from build123d import *

# Parameters (mm, degrees)
BOSS_EXTRUDE1_DEPTH       = 80
SKETCH2_W                 = 60
SKETCH2_H                 = 80
BOSS_EXTRUDE6_DEPTH       = 10
CUT_EXTRUDE3_DEPTH        = 149
BOSS_EXTRUDE7_DEPTH       = 20
SKETCH11_W                = 100
SKETCH11_H                = 80
CUT_EXTRUDE4_DEPTH        = 20
CUT_EXTRUDE5_DEPTH        = 20
SKETCH14_W                = 24.037008503
SKETCH14_H                = 50
CUT_EXTRUDE6_DEPTH        = 29
SKETCH15_W                = 46.666666667
SKETCH15_H                = 50
CUT_EXTRUDE7_DEPTH        = 29
SKETCH16_W                = 20
SKETCH16_H                = 30
BOSS_EXTRUDE8_DEPTH       = 70
BOSS_EXTRUDE10_DEPTH      = 30
SKETCH21_W                = 43.205783384
SKETCH21_H                = 74.052806938
CUT_EXTRUDE9_DEPTH        = 30
SKETCH22_W                = 30
SKETCH22_H                = 20
CUT_EXTRUDE10_DEPTH       = 30
BOSS_EXTRUDE11_DEPTH      = 30
BOSS_EXTRUDE12_DEPTH      = 40
BOSS_EXTRUDE12_DEPTH_BACK = 30
SKETCH25_W                = 50
SKETCH25_H                = 20
BOSS_EXTRUDE13_DEPTH      = 60
BOSS_EXTRUDE16_DEPTH      = 50
BOSS_EXTRUDE17_DEPTH      = 20


with BuildPart() as part:
    # Sketch1 → Boss-Extrude1 (new body)
    with BuildSketch(Plane(origin=(0, 0, 0), x_dir=(1, 0, 0), z_dir=(0, 1, 0))):
        Polygon((0, 0), (0, 60), (40, 60), (40, 30), (30, 30), (30, 20), align=None)
    extrude(amount=BOSS_EXTRUDE1_DEPTH)

    # Sketch2 → Boss-Extrude6 (add)
    with BuildSketch(Plane.ZY):
        with Locations((-30, 40)):
            Rectangle(SKETCH2_W, SKETCH2_H)
        Polygon((40, 0), (0, 0), (0, 80), (20, 50), (40, 50), align=None)
    extrude(amount=-BOSS_EXTRUDE6_DEPTH)

    # Sketch8 → Cut-Extrude3 (cut)
    with BuildSketch(Plane(origin=(18.823529412, 18.823529412, 28.235294118), x_dir=(0.874474632, -0.269069118, -0.403603676), z_dir=(0.48507125, 0.48507125, 0.727606875))):
        Polygon((-21.525529408, 30.508510792), (12.780783086, 41.602514717), (12.780783086, 77.658027472), (-21.525529408, 66.564023547), align=None)
    extrude(amount=CUT_EXTRUDE3_DEPTH, mode=Mode.SUBTRACT)

    # Sketch10 → Boss-Extrude7 (add)
    with BuildSketch(Plane(origin=(18.823529412, 18.823529412, 28.235294118), x_dir=(0.874474632, -0.269069118, -0.403603676), z_dir=(0.48507125, 0.48507125, 0.727606875))):
        Polygon((-21.525529408, 30.508510792), (12.780783086, 41.602514717), (12.780783086, 77.658027472), (-21.525529408, 66.564023547), align=None)
    extrude(amount=-BOSS_EXTRUDE7_DEPTH)

    # Sketch11 → Cut-Extrude4 (cut)
    with BuildSketch(Plane.ZY):
        with Locations((-10, 40)):
            Rectangle(SKETCH11_W, SKETCH11_H)
    extrude(amount=CUT_EXTRUDE4_DEPTH, mode=Mode.SUBTRACT)

    # Sketch12 → Cut-Extrude5 (cut)
    with BuildSketch(Plane(origin=(0, 50, 0), x_dir=(1, 0, 0), z_dir=(0, 1, 0))):
        Polygon((0, -20), (10, -13.333333333), (10, -40), (0, -40), align=None)
    extrude(amount=CUT_EXTRUDE5_DEPTH, mode=Mode.SUBTRACT)

    # Sketch14 → Cut-Extrude6 (cut)
    with BuildSketch(Plane(origin=(0, 0, 0), x_dir=(0.832050294, 0, -0.554700196), z_dir=(0.554700196, 0, 0.832050294))):
        with Locations((24.037008504, 25)):
            Rectangle(SKETCH14_W, SKETCH14_H)
    extrude(amount=CUT_EXTRUDE6_DEPTH, mode=Mode.SUBTRACT)

    # Sketch15 → Cut-Extrude7 (cut)
    with BuildSketch(Plane(origin=(10, 0, 0), x_dir=(0, 0, -1), z_dir=(1, 0, 0))):
        with Locations((-16.666666666, 25)):
            Rectangle(SKETCH15_W, SKETCH15_H)
    extrude(amount=CUT_EXTRUDE7_DEPTH, mode=Mode.SUBTRACT)

    # Sketch16 → Boss-Extrude8 (add)
    with BuildSketch(Plane(origin=(0, 70, 0), x_dir=(1, 0, 0), z_dir=(0, 1, 0))):
        with Locations((50, 45)):
            Rectangle(SKETCH16_W, SKETCH16_H)
    extrude(amount=-BOSS_EXTRUDE8_DEPTH)

    # Sketch17 → Boss-Extrude10 (add)
    with BuildSketch(Plane(origin=(0, 0, -60), x_dir=(-1, 0, 0), z_dir=(0, 0, -1))):
        Polygon((-80, 10), (-80, 0), (-60, 0), (-60, 70), (-100, 10), align=None)
    extrude(amount=-BOSS_EXTRUDE10_DEPTH)

    # Sketch21 → Cut-Extrude9 (cut)
    with BuildSketch(Plane.XY.offset(-30)):
        with Locations((81.602891692, 32.973596531)):
            Rectangle(SKETCH21_W, SKETCH21_H)
    extrude(amount=-CUT_EXTRUDE9_DEPTH, mode=Mode.SUBTRACT)

    # Sketch22 → Cut-Extrude10 (cut)
    with BuildSketch(Plane.XY.offset(-30)):
        with Locations((45, 10)):
            Rectangle(SKETCH22_W, SKETCH22_H)
    extrude(amount=-CUT_EXTRUDE10_DEPTH, mode=Mode.SUBTRACT)

    # Sketch23 → Boss-Extrude11 (add)
    with BuildSketch(Plane.XY.offset(-30)):
        Polygon((60, 70), (100, 30), (80, 30), (80, 20), (60, 20), align=None)
    extrude(amount=-BOSS_EXTRUDE11_DEPTH)

    # Sketch24 → Boss-Extrude12 (add, two sides)
    with BuildSketch(Plane.XY.offset(-30)) as boss_extrude12_sk:
        Polygon((100, 30), (120, 10), (120, 0), (80, 0), (80, 30), align=None)
    extrude(amount=BOSS_EXTRUDE12_DEPTH)
    extrude(boss_extrude12_sk.sketch, amount=-BOSS_EXTRUDE12_DEPTH_BACK)

    # Sketch25 → Boss-Extrude13 (add)
    with BuildSketch(Plane(origin=(0, 0, -60), x_dir=(-1, 0, 0), z_dir=(0, 0, -1))):
        with Locations((-55, 10)):
            Rectangle(SKETCH25_W, SKETCH25_H)
    extrude(amount=-BOSS_EXTRUDE13_DEPTH)

    # Sketch28 → Boss-Extrude16 (add)
    with BuildSketch(Plane(origin=(0, 0, 0), x_dir=(-1, 0, 0), z_dir=(0, -1, 0))):
        Polygon((-10, 6.666666667), (-30, 20), (-10, -6.666666667), align=None)
        Polygon((-10, -6.666666667), (-30, 20), (-30, 0), (-30, -20), (-10, -40), align=None)
    extrude(amount=-BOSS_EXTRUDE16_DEPTH)

    # Sketch29 → Boss-Extrude17 (add)
    with BuildSketch(Plane(origin=(30, 0, 0), x_dir=(0, 0, -1), z_dir=(1, 0, 0))):
        Polygon((0, 50), (20, 50), (20, 80), align=None)
    extrude(amount=-BOSS_EXTRUDE17_DEPTH)


solid = part.part
Could you check a few things on this model? Use its own coordinates, in mm. A direction names the side the tool comes from. Give positions to 0.01 mm unless a question says otherwise; leave off trailing zeros. Order: outer loops, then holes, each group sorted by start corner. A loop starts at its lowest first (then second) coordinate and runs counter-clockwise, first axis right, second up.
Item 1: I need wall thicknesses on line 1 (X direction, y = 41.5, z = -10); line 2 (Z direction, x = 75, y = 22.5); line 3 (Z direction, x = 102.5, y = 23). Which ranges of each line are inside material? Lowest first, please.
Item 2: For faces 4 (the face through (30, 41, -5)), 5 (the face through (50, 70, -45)), 6 (the face through (15, 50, 20)), 7 (the face through (96, 15, 10)), 8 (the face through (55, 10, 0)), which set-ups out of +Z, -Z, +X, -X, +Y, -Y let a thin tool reach every point of the face, with its end or its side?
Item 3: If we section it at A-A, the plane z = 1.5: Write out the boundary of the cut face in (x, y), plus the area to 3 significant figures.
Item 4: If we section it at C-C, the plane z = -12: Write out the boundary of the cut face in (x, y), plus the area to 3 significant figures.
Item 5: If we section it at B-B, the plane y = 41.5: Write out the boundary of the cut face in (x, z), plus the area to 4 significant figures.
Item 6: If we mould it in two halves opening along X, with no side actions, what happens to faces 1 (the face through (40, 75, -45)), 2 (the face through (48, 32, -60)), 3 (the face through (58, 44, -30))? For each: pulls with the +X half, pulls with the -X half, needs draft (parallel to the pull), parting line crosses it, or undercut.
Item 7: If we section it at D-D, the plane x = 13.5: Write out the boundary of the cut face in (y, z).
Item 8: I'm going to push flat-ended pins straight in: pin 1 (12 mm diameter, centred on x = 53.5, z = 10.5, fed in from -Y); pin 2 (5 mm diameter, centred on y = 14, z = 18.5, fed in from +X); pin 3 (3 mm diameter, centred on y = 74.5, z = -41, fed in from +X); pin 4 (15 mm diameter, centred on x = 22, z = 14, fed in from +Y). Where does each tip first touch, or does it pass through?
Values:
1. line 1: x = 0 to 30
1. line 2: z = -60 to -30
1. line 3: z = -60 to 10
2. face 4: +Z, +Y
2. face 5: +Z, -Z, +X, +Y
2. face 6: +Z, +X, +Y
2. face 7: +Z, +X, +Y, -Y
2. face 8: +Z, +Y, -Y
3. outline: (0, 0) - (30, 0) - (30, 50) - (27.75, 50) - (0, 77.75) - close; (80, 0) - (120, 0) - (120, 10) - (100, 30) - (80, 30) - close
3. area: 2,890 mm2
4. outline: (0, 0) - (120, 0) - (120, 10) - (100, 30) - (80, 30) - (80, 20) - (30, 20) - (30, 68) - (18, 80) - (0, 80) - close
4. area: 4,330 mm2
5. outline: (0, -60) - (88.5, -60) - (88.5, -30) - (30, -30) - (30, 20) - (10, 40) - (0, 40) - close
5. area: 4,555 mm2
6. face 1: pulls with the +X half
6. face 2: needs draft
6. face 3: undercut
7. outline: (0, -60) - (80, -60) - (80, -9) - (50, 11) - (50, 36.5) - (0, 36.5) - close
8. pin 1: passes through
8. pin 2: stops at x = 30
8. pin 3: stops at x = 40
8. pin 4: stops at y = 50.52
